The figure shows three views and two pictorial views of one solid part (mm, origin at its lowest corner). Answer the questions. A direction names the side the tool comes from. Give positions to 0.01 mm unless a question says otherwise; leave off trailing zeros. Loops run counter-clockwise (first coordinate to the right, second up) from the corner with the lowest first, then second, coordinate; pieces in that order, holes last.
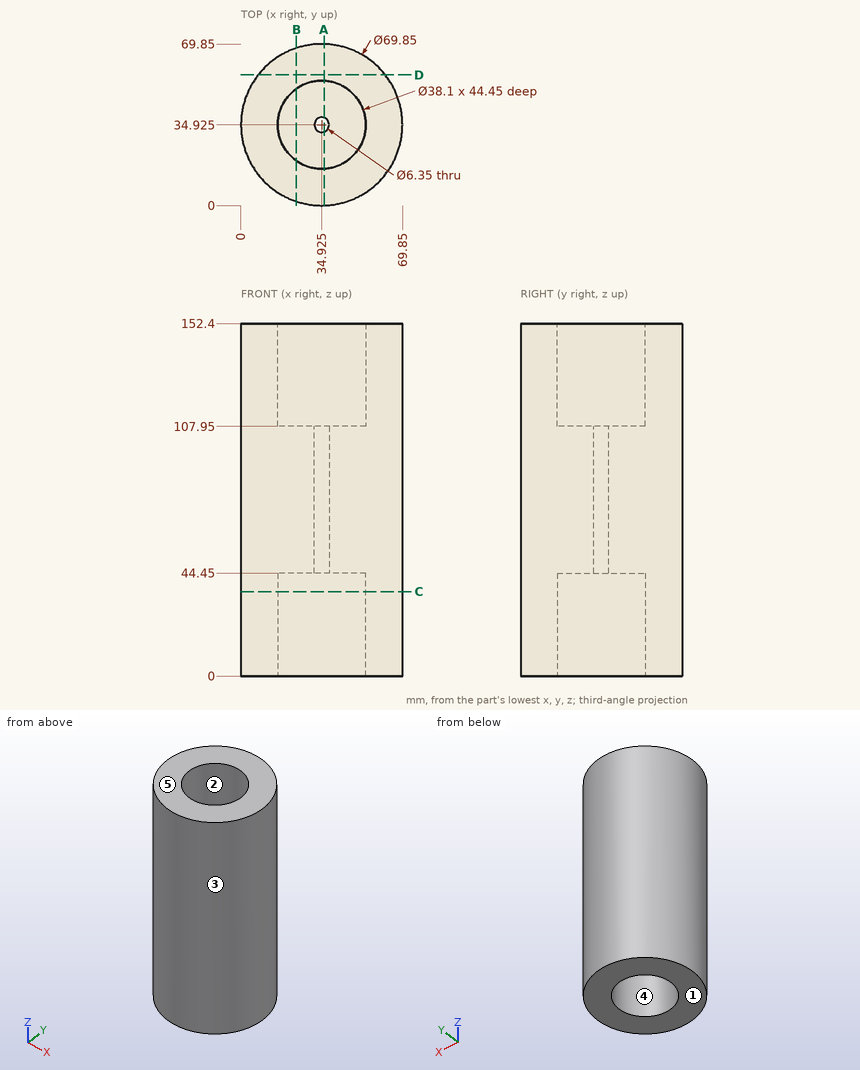
Q1. Given pin 1 (7.5 mm diameter, centred on x = 34.925, y = 34.925, fed in from -Z); pin 2 (4 mm diameter, centred on y = 45.5, z = 126.5, fed in from +X); pin 3 (6 mm diameter, centred on x = 47.5, y = 25.5, fed in from +Z), each flat-ended and moving along its own axis, determine where each tip first touches the part or whether it passes through.
Q2. Section A-A on x = 36 is taken. Give the vertices of the cut face in (y, z).
Q3. Consider line 1 along Z through (x, y) = (51.5, 34); line 2 along X through (y, z) = (44.5, 7.5); line 3 along X through (y, z) = (42.5, 144.5). Determine where each line is inside the solid, lowest interval first.
Q4. Which of the six approach directions +Z, -Z, +X, -X, +Y, -Y give full straight-line access (tool end or side, diameter ignored) to the marked faces 4 and 5?
Q5. Section D-D on y = 56.5 is taken. Give the vertices of the cut face in (x, z), plus the area to 3 significant figures.
Q6. Section C-C on z = 36.5 is taken. Give the vertices of the cut face in (x, y) (3 decimals), plus the area to 3 significant figures.
Q7. Determine the mould class of the marked faces 1, 2 and 3 for opening direction Y: +Y half, -Y half, draft (parallel to the pull), parting line (faces both ways), or undercut.
Q8. Section B-B on x = 24 is taken. Give the vertices of the cut face in (y, z), plus the area to 3 significant figures.
Check result:
1. pin 1: stops at z = 44.45
1. pin 2: stops at x = 68.78
1. pin 3: stops at z = 107.95
2. outline: (0.02, 0) - (15.91, 0) - (15.91, 44.45) - (31.94, 44.45) - (31.94, 107.95) - (15.91, 107.95) - (15.91, 152.4) - (0.02, 152.4) - close; (37.91, 44.45) - (53.94, 44.45) - (53.94, 0) - (69.83, 0) - (69.83, 152.4) - (53.94, 152.4) - (53.94, 107.95) - (37.91, 107.95) - close
3. line 1: z = 44.45 to 107.95
3. line 2: x = 1.34 to 18.46, 51.39 to 68.51
3. line 3: x = 0.83 to 17.45, 52.4 to 69.02
4. face 4: -Z
4. face 5: +Z, +X, -X, +Y, -Y
5. outline: (7.46, 0) - (62.39, 0) - (62.39, 152.4) - (7.46, 152.4) - close
5. area: 8,370 mm2
6. outline: circle Ø69.85 at (34.925, 34.925); hole circle Ø38.1 at (34.925, 34.925)
6. area: 2,690 mm2
7. face 1: draft
7. face 2: undercut
7. face 3: parting line
8. outline: (1.75, 0) - (19.32, 0) - (19.32, 44.45) - (50.53, 44.45) - (50.53, 0) - (68.1, 0) - (68.1, 152.4) - (50.53, 152.4) - (50.53, 107.95) - (19.32, 107.95) - (19.32, 152.4) - (1.75, 152.4) - close
8. area: 7,340 mm2
